Could you check a few things on this model? Use its own coordinates, in mm. Face numbers are marked on the shaded views. A direction names the side the tool comes from. Give positions to 0.01 mm unless a question says otherwise; leave off trailing zeros. Loops run counter-clockwise (first coordinate to the right, second up) from the corner with the lowest first, then second, coordinate; pieces in that order, holes last. Notation, with made-up numbers: (-14.75, 48) - (-2.75, 48) arc R22 ccw to (-2.75, 61) - close; hole circle Ø6 at (-4.5, 59). An arc over 180 degrees is marked (long way). One line per item, written item: value. Start each with the question number.
Q1. For the marked faces 1, 2 and 3, which set-ups out of +Z, -Z, +X, -X, +Y, -Y let a thin tool reach every point of the face, with its end or its side?
Q2. I'm going to push flat-ended pins straight in: P1, Ø3, axis at x = -73.5, y = 25, coming from the -Z side; P2, Ø3, axis at y = 21, z = 1.5, coming from the +X side; P3, Ø3, axis at y = 6, z = 3.5, coming from the +X side; P4, Ø1, axis at y = 11, z = 1.5, coming from the +X side. Where does each tip first touch, or does it pass through?
Q3. I want a section at C-C (z = 0.75). Please give me the cut outline in (x, y) (3 decimals), then the cut area to 3 significant figures.
Q4. If we mould it in two halves opening along X, with no side actions, what happens to the marked faces 4, 5 and 6? For each: released by +X, released by -X, zero draft, split by the parting line, or undercut.
Q5. I want a section at D-D (x = -14.5). Please give me the cut outline in (y, z), then the cut area to 3 significant figures.
Q6. I want a section at B-B (y = 11). Please give me the cut outline in (x, z), then the cut area to 3 significant figures.
Q7. I want a section at A-A (x = -60.5). Please give me the cut outline in (y, z).
Q8. If I drill on line 1 (Y direction, x = 5, z = 2.5); line 2 (X direction, y = 15, z = 1.8); line 3 (Y direction, x = -60, z = 3.9), over which ranges is the centre line in solid material (lowest first)? Write a range as from..to.
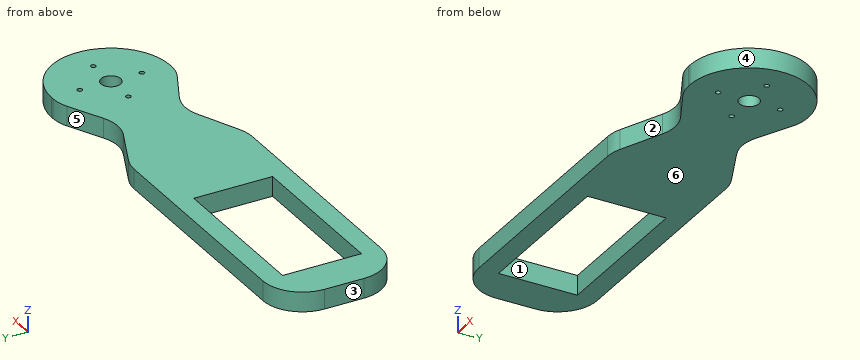
```python
from build123d import *

# Parameters (mm, degrees)
SKETCH1_R           = 2.5
SKETCH1_R_2         = 0.635
SKETCH1_W           = 40
SKETCH1_H           = 20
BOSS_EXTRUDE1_DEPTH = 5
CUT_EXTRUDE1_DEPTH  = 5
FILLET1_R           = 10
FILLET2_R           = 10


with BuildPart() as part:
    # Sketch1 → Boss-Extrude1 (new body)
    with BuildSketch(Plane.XY):
        with BuildLine():
            Line((5, -0.042056462), (-100, -0.042056462))
            Line((-100, -0.042056462), (-100, 29.957943538))
            Line((-100, 29.957943538), (5, 29.957943538))
            ThreePointArc((5, 29.957943538), (20, 14.957943538), (5, -0.042056462))
        make_face()
        with Locations((5, 14.957943538)):
            Circle(SKETCH1_R, mode=Mode.SUBTRACT)
        with Locations((5, 22.832946838)):
            Circle(SKETCH1_R_2, mode=Mode.SUBTRACT)
        with Locations((-2.8750033, 14.957943538)):
            Circle(SKETCH1_R_2, mode=Mode.SUBTRACT)
        with Locations((12.8750033, 14.957943538)):
            Circle(SKETCH1_R_2, mode=Mode.SUBTRACT)
        with Locations((5, 7.082940238)):
            Circle(SKETCH1_R_2, mode=Mode.SUBTRACT)
        with Locations((-70, 14.957943538)):
            Rectangle(SKETCH1_W, SKETCH1_H, mode=Mode.SUBTRACT)
    extrude(amount=BOSS_EXTRUDE1_DEPTH)

    # Sketch2 → Cut-Extrude1 (cut)
    with BuildSketch(Plane.XY.offset(5)):
        with BuildLine():
            Line((-28.071470169, 29.107121554), (-17.302448086, 24.356082399))
            ThreePointArc((-17.302448086, 24.356082399), (-13.025291719, 23.508158967), (-8.793910065, 24.560988505))
            Line((-8.793910065, 24.560988505), (-0.11145618, 28.902215448))
            ThreePointArc((-0.11145618, 28.902215448), (2.06315057, 29.690433433), (4.360679775, 29.957943538))
            Line((4.360679775, 29.957943538), (-32.107872235, 29.957943538))
            ThreePointArc((-32.107872235, 29.957943538), (-30.04532286, 29.742926424), (-28.071470169, 29.107121554))
        make_face()
        with BuildLine():
            Line((-28.071470169, 0.808765522), (-17.302448086, 5.559804676))
            ThreePointArc((-17.302448086, 5.559804676), (-13.025291719, 6.407728109), (-8.793910065, 5.354898571))
            Line((-8.793910065, 5.354898571), (-0.11145618, 1.013671628))
            ThreePointArc((-0.11145618, 1.013671628), (2.06315057, 0.225453643), (4.360679775, -0.042056462))
            Line((4.360679775, -0.042056462), (-32.107872235, -0.042056462))
            ThreePointArc((-32.107872235, -0.042056462), (-30.04532286, 0.172960652), (-28.071470169, 0.808765522))
        make_face()
    extrude(amount=-CUT_EXTRUDE1_DEPTH, mode=Mode.SUBTRACT)

    # Fillet1
    fillet1_edges = [part.edges().sort_by_distance(p)[0] for p in [
        (-100, 29.957943538, 2.5),
    ]]
    fillet(fillet1_edges, radius=FILLET1_R)

    # Fillet2
    fillet2_edges = [part.edges().sort_by_distance(p)[0] for p in [
        (-100, -0.042056462, 2.5),
    ]]
    fillet(fillet2_edges, radius=FILLET2_R)


solid = part.part
```
Worked answers:
1. face 1: +Z, -Z
1. face 2: +Z, -Z, -Y
1. face 3: +Z, -Z, -X, +Y, -Y
2. P1: stops at z = 0
2. P2: stops at x = 19.3
2. P3: stops at x = 18.01
2. P4: stops at x = 19.6
3. outline: (-100, 9.958) arc R10 ccw to (-90, -0.042) - (-32.108, -0.042) arc R10 ccw to (-28.071, 0.809) - (-17.302, 5.56) arc R10 cw to (-8.794, 5.355) - (-0.111, 1.014) arc R10 ccw to (4.361, -0.042) - (5, -0.042) arc R15 ccw to (5, 29.958) - (4.361, 29.958) arc R10 ccw to (-0.111, 28.902) - (-8.794, 24.561) arc R10 cw to (-17.302, 24.356) - (-28.071, 29.107) arc R10 ccw to (-32.108, 29.958) - (-90, 29.958) arc R10 ccw to (-100, 19.958) - close; hole (-90, 4.958) - (-50, 4.958) - (-50, 24.958) - (-90, 24.958) - close; hole circle Ø1.27 at (-2.875, 14.958); hole circle Ø5 at (5, 14.958); hole circle Ø1.27 at (5, 7.083); hole circle Ø1.27 at (5, 22.833); hole circle Ø1.27 at (12.875, 14.958)
3. area: 2,400 mm²
4. face 4: released by +X
4. face 5: undercut
4. face 6: zero draft
5. outline: (6.33, 0) - (23.58, 0) - (23.58, 5) - (6.33, 5) - close
5. area: 86.2 mm²
6. outline: (-100, 0) - (-90, 0) - (-90, 5) - (-100, 5) - close; (-50, 0) - (19.47, 0) - (19.47, 5) - (-50, 5) - close
6. area: 397 mm²
7. outline: (-0.04, 0) - (4.96, 0) - (4.96, 5) - (-0.04, 5) - close; (24.96, 0) - (29.96, 0) - (29.96, 5) - (24.96, 5) - close
8. line 1: y = -0.04..6.45, 7.72..12.46, 17.46..22.2, 23.47..29.96
8. line 2: x = -100..-90, -50..-3.51, -2.24..2.5, 7.5..12.24, 13.51..20
8. line 3: y = -0.04..4.96, 24.96..29.96
